Check sheet for the modelled part. Datum: model origin and axes. Units: mm. A direction names the side the tool comes from. Round coordinates to 2 decimals unless told otherwise and drop trailing zeros. Order: outer loops, then holes, each group sorted by start corner. A loop starts at its lowest first (then second) coordinate and runs counter-clockwise, first axis right, second up.
```python
from build123d import *

# Parameters (mm, degrees)
ESQUISSE2_R                  = 6
ESQUISSE2_R_2                = 1.6
BOSS_EXTRU_1_DEPTH           = 2.7
ESQUISSE3_R                  = 1.6
ENL_V_MAT_EXTRU_1_DEPTH      = 69.646121522
R_P_TITION_CIRCULAIRE1_COUNT = 6


with BuildPart() as part:
    # Esquisse2 → Boss.-Extru.1 (new body)
    with BuildSketch(Plane(origin=(0, 0, 0), x_dir=(1, 0, 0), z_dir=(0, 1, 0))):
        with BuildLine():
            Line((-17, -48), (-5, -48))
            ThreePointArc((-5, -48), (24.685348475, -37.719757236), (41.655172414, -11.28250358))
            ThreePointArc((41.655172414, -11.28250358), (43.286450296, -7.752943214), (46.140625, -5.112384435))
            ThreePointArc((46.140625, -5.112384435), (49, 0), (46.140625, 5.112384435))
            ThreePointArc((46.140625, 5.112384435), (43.286450296, 7.752943214), (41.655172414, 11.28250358))
            ThreePointArc((41.655172414, 11.28250358), (24.685348475, 37.719757236), (-5, 48))
            Line((-5, 48), (-17, 48))
            ThreePointArc((-17, 48), (-20.20664932, 47.071232606), (-22.420554861, 44.572466714))
            ThreePointArc((-22.420554861, 44.572466714), (-32.460451204, 0), (-22.420554861, -44.572466714))
            ThreePointArc((-22.420554861, -44.572466714), (-20.20664932, -47.071232606), (-17, -48))
        make_face()
        with Locations(Location((-5, 0, 0), (0, 0, 90))):
            Circle(ESQUISSE2_R, mode=Mode.SUBTRACT)
        with Locations(Location((24.69848481, 29.69848481, 0), (0, 0, 90))):
            Circle(ESQUISSE2_R_2, mode=Mode.SUBTRACT)
        with Locations(Location((24.69848481, -29.69848481, 0), (0, 0, 90))):
            Circle(ESQUISSE2_R_2, mode=Mode.SUBTRACT)
        with BuildLine():
            Line((-17, 44.1), (-11, 44.1))
            ThreePointArc((-11, 44.1), (-8.9, 42), (-11, 39.9))
            Line((-11, 39.9), (-17, 39.9))
            ThreePointArc((-17, 39.9), (-19.1, 42), (-17, 44.1))
        make_face(mode=Mode.SUBTRACT)
        with BuildLine():
            Line((43, 2.1), (37, 2.1))
            ThreePointArc((37, 2.1), (34.9, 0), (37, -2.1))
            Line((37, -2.1), (43, -2.1))
            ThreePointArc((43, -2.1), (45.1, 0), (43, 2.1))
        make_face(mode=Mode.SUBTRACT)
        with BuildLine():
            Line((-17, -44.1), (-11, -44.1))
            ThreePointArc((-11, -44.1), (-8.9, -42), (-11, -39.9))
            Line((-11, -39.9), (-17, -39.9))
            ThreePointArc((-17, -39.9), (-19.1, -42), (-17, -44.1))
        make_face(mode=Mode.SUBTRACT)
    extrude(amount=BOSS_EXTRU_1_DEPTH)

    # Esquisse3 → Enl_v. mat.-Extru.1 (cut, through all)
    with BuildSketch(Plane(origin=(0, 0, 0), x_dir=(1, 0, 0), z_dir=(0, 1, 0))):
        with Locations(Location((2, 15.5, 0), (0, 0, 90))):
            Circle(ESQUISSE3_R)
    enl_v_mat_extru_1 = extrude(amount=ENL_V_MAT_EXTRU_1_DEPTH, mode=Mode.SUBTRACT)

    # R_p_tition circulaire1: Enl_v. mat.-Extru.1 ×6 about axis
    r_p_tition_circulaire1_axis = Axis((2, 0, 0), (0, 1, 0))
    for i in range(1, R_P_TITION_CIRCULAIRE1_COUNT):
        add(enl_v_mat_extru_1.rotate(r_p_tition_circulaire1_axis, i * 360 / R_P_TITION_CIRCULAIRE1_COUNT), mode=Mode.SUBTRACT)


solid = part.part
```
Item 1: Sectioned sample at D-D (y = 2.15). State how many separate pieces and enclosed holes the cut face has, and give its area (3 significant figures).
Answer:
separate pieces: 1
enclosed holes: 12
area: 5,660 mm2
Item 2: Scan lines: line 1 along X through (y, z) = (2, 0); line 2 along Z through (x, y) = (-10, 1.65); line 3 along X through (y, z) = (1.35, 7.75). Record each from-to range of solid material in increasing order.
Answer:
line 1: x = -32.46 to -11, 1 to 34.9, 45.1 to 49
line 2: z = -48 to -43.85, -40.15 to -8.48, -7.02 to -3.32, 3.32 to 7.02, 8.48 to 40.15, 43.85 to 48
line 3: x = -32.17 to -13.02, -9.82 to 13.82, 17.02 to 43.29
Item 3: Sectioned sample at C-C (z = -15.5). Record the cut outline in (x, y).
Answer:
outline: (-31.3, 0) - (0.4, 0) - (0.4, 2.7) - (-31.3, 2.7) - close; (3.6, 0) - (40.43, 0) - (40.43, 2.7) - (3.6, 2.7) - close
Item 4: Access from +Z, -Z, +X, -X, +Y, -Y to the whole of each face (thin tool, end or side, straight path). Record for faces 5 (the cylindrical face through (-8.9, 1.3, -42)), 6 (the flat face through (-11, 1, 48)).
Answer:
face 5: +Y, -Y
face 6: +Z, +X, -X, +Y, -Y
Item 5: Go/stop test with a flat-tipped pin: P1, Ø1, axis at x = 22, y = 1, coming from the +Z side. Record where the tip stops, or that it passes through.
Answer:
P1: stops at z = 40.02
Item 6: Release check for a two-part mould opening along X. For faces 1 (the cylindrical face through (24.332, 1.331, 37.995)), 2 (the cylindrical face through (-20.167, 1.331, -47.096)), 3 (the flat face through (-14, 1, 39.9)), 4 (the flat face through (8, 2.7, -1)) record: released by +X, released by -X, zero draft, split by the parting line, or undercut.
Answer:
face 1: released by +X
face 2: released by -X
face 3: undercut
face 4: zero draft
Item 7: Sectioned sample at B-B (x = -1.5). Record the cut outline in (y, z), and give its area (3 significant figures).
Answer:
outline: (0, -47.87) - (2.7, -47.87) - (2.7, -4.87) - (0, -4.87) - close; (0, 4.87) - (2.7, 4.87) - (2.7, 47.87) - (0, 47.87) - close
area: 232 mm2
Item 8: Sectioned sample at A-A (z = 0). Record the cut outline in (x, y).
Answer:
outline: (-32.46, 0) - (-11, 0) - (-11, 2.7) - (-32.46, 2.7) - close; (1, 0) - (34.9, 0) - (34.9, 2.7) - (1, 2.7) - close; (45.1, 0) - (49, 0) - (49, 2.7) - (45.1, 2.7) - close
